Source: three-view drawing plus pictorial views. Frame: mm from the lowest corner of the part. Coordinates: 2 decimals unless noted, no trailing zeros. Order: outer loops, then holes, each group sorted by start corner. A loop starts at its lowest first (then second) coordinate and runs counter-clockwise, first axis right, second up. Notation, with made-up numbers: (18, 22) - (48, 22) arc R18 cw to (48, 48) - close; hole circle Ø2 at (89, 58). An arc over 180 degrees is marked (long way). One line per question, with ' | ' between items.
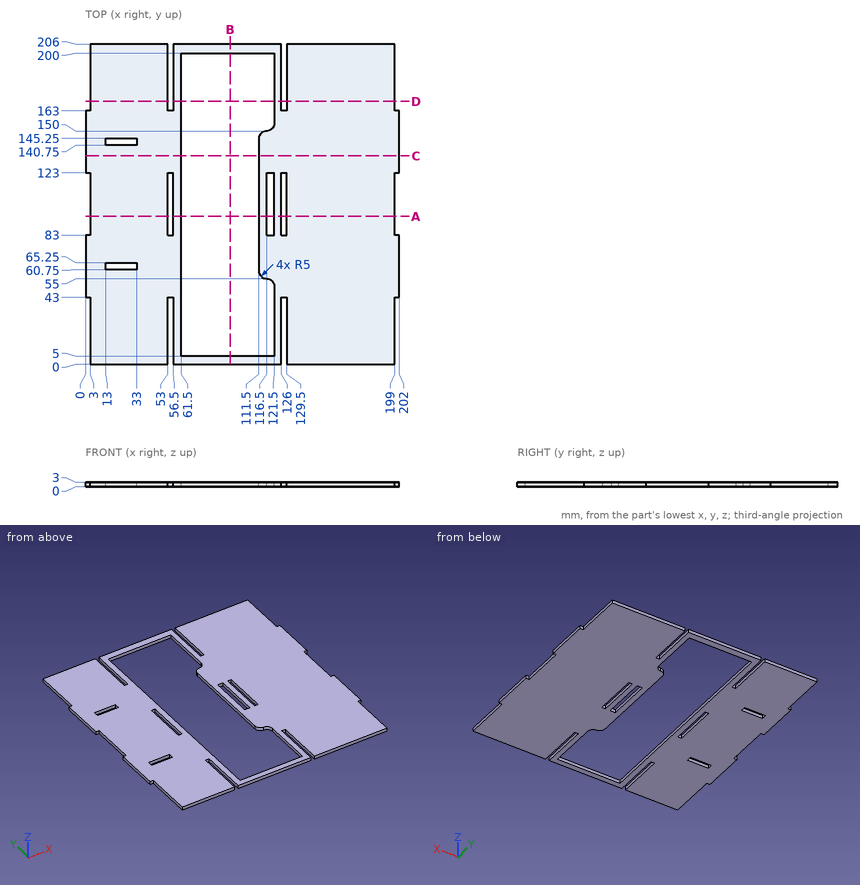
Item 1: Section D-D on y = 169. Return the cut outline in (x, z), and give its area (3 significant figures).
Data:
outline: (3, 0) - (53, 0) - (53, 3) - (3, 3) - close; (56.5, 0) - (61.5, 0) - (61.5, 3) - (56.5, 3) - close; (121.5, 0) - (126, 0) - (126, 3) - (121.5, 3) - close; (129.5, 0) - (199, 0) - (199, 3) - (129.5, 3) - close | area: 387 mm^2
Item 2: Section A-A on y = 95. Return the cut outline in (x, z).
Data:
outline: (3, 0) - (53, 0) - (53, 3) - (3, 3) - close; (56.5, 0) - (61.5, 0) - (61.5, 3) - (56.5, 3) - close; (111.5, 0) - (116.5, 0) - (116.5, 3) - (111.5, 3) - close; (121.5, 0) - (126, 0) - (126, 3) - (121.5, 3) - close; (129.5, 0) - (199, 0) - (199, 3) - (129.5, 3) - close
Item 3: Section C-C on y = 134. Return the cut outline in (x, z).
Data:
outline: (0, 0) - (61.5, 0) - (61.5, 3) - (0, 3) - close; (111.5, 0) - (202, 0) - (202, 3) - (111.5, 3) - close
Item 4: Ray query, line 1 (X direction, y = 111, z = 0.85); line 2 (X direction, y = 62, z = 0.35); line 3 (Y direction, x = 26, z = 2.05). Return the intervals inside material, ascending.
Data:
line 1: 3 to 53, 56.5 to 61.5, 111.5 to 116.5, 121.5 to 126, 129.5 to 199 | line 2: 0 to 13, 33 to 61.5, 111.5 to 202 | line 3: 0 to 60.75, 65.25 to 140.75, 145.25 to 206
Item 5: Section B-B on x = 93. Return the cut outline in (y, z), and give its area (3 significant figures).
Data:
outline: (0, 0) - (5, 0) - (5, 3) - (0, 3) - close; (200, 0) - (206, 0) - (206, 3) - (200, 3) - close | area: 33.0 mm^2
Item 6: Contact query for flat-ended pins moving along their axis: P1, Ø0.9, axis at x = 1, z = 1.5, coming from the +Y side; P2, Ø1, axis at y = 183.5, z = 2, coming from the -X side. Output: stop coordinate, or through.
Data:
P1: y = 163 | P2: x = 3
